Source: CAD feature listing. Evaluate the final solid. Frame: model axes, mm. Face numbers are marked on the shaded views. A direction names the side the tool comes from. Round coordinates to 2 decimals unless told otherwise and drop trailing zeros. Loops run counter-clockwise (first coordinate to the right, second up) from the corner with the lowest first, then second, coordinate; pieces in that order, holes last. Notation, with made-up numbers: M 65.5,56.5 L 79.5,56.5 A26 ccw 79.5,74.5 Z; hole C -19,9.25 d4. An arc over 180 degrees is marked long. Write each question's results on one line, items separated by ' | '. Start each with the question number.
1. Contact query for a flat-ended pin moving along its axis: pin 1 Ø4 at (x, z) = (-1, -13.5) entering from -Y. Output: stop coordinate, or through.
2. Set-up query: the marked faces 4 and 5. Return all of +Z, -Z, +X, -X, +Y, -Y with unobstructed straight access to the full face (end or side cutting, diameter ignored); none if empty.
3. Section C-C on y = 7.5. Output: boundary loops of the cut face in (x, z), and give its area (3 significant figures).
4. Ray query, line 1 (Z direction, x = 1.5, y = 0); line 2 (X direction, y = 10.75, z = -15.5); line 3 (Z direction, x = -6, y = 2.25). Return the intervals inside material, ascending.
5. Section A-A on z = -15.5. Output: boundary loops of the cut face in (x, y).
6. Draft query along Z for the marked faces 1, 2 and 3. Return one class per face: released by +Z, released by -Z, zero draft, split by the parting line, or undercut.
7. Section D-D on x = -4.5. Output: boundary loops of the cut face in (y, z).
8. Section B-B on x = 0. Output: boundary loops of the cut face in (y, z), and give its area (3 significant figures).
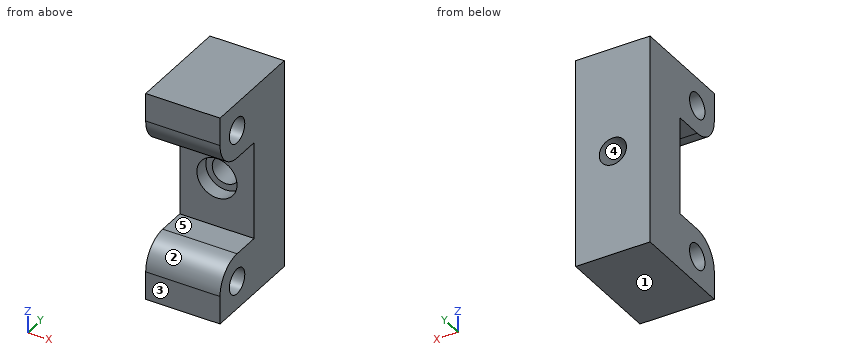
Autodesk Inventor part; units mm, degrees
ref_plane "Work Plane1" through (0, 5.5, 0) normal (0, 1, 0) x (-1, 0, 0)
ref_plane "YZ Plane" through (0, 0, 0) normal (1, 0, 0) x (0, 1, 0)
ref_plane "XY Plane" through (0, 0, 0) normal (0, 0, 1) x (1, 0, 0)
sketch "Sketch3" plane through (0, 0, 0) normal (1, 0, 0) x (0, 1, 0)
  circle A0 centre (0, 0) radius 5.65 construction
  line L0 (-5.65, 0) -> (-5.65, 5.65)
  line L1 (0, -5.65) -> (5.65, -5.65)
  arc A1 (-5.65, 0) -> (0, -5.65) centre (0, 0) ccw
  line L2 (-5.65, 5.65) -> (5.65, 5.65)
  line L3 (5.65, -15.5) -> (-5.65, -15.5) construction
  line L4 (5.65, 5.65) -> (15.65, 5.65)
  line L5 (15.65, 5.65) -> (15.65, -15.5)
  line L6 (5.65, -5.65) -> (5.65, -15.5)
  line L7 (15.65, -15.5) -> (5.65, -15.5) construction
  circle A2 centre (0, 0) radius 2.55
  line L8 (-5.65, -31) -> (-5.65, -36.65)
  arc A3 (0, -25.35) -> (-5.65, -31) centre (0, -31) ccw
  line L9 (0, -25.35) -> (5.65, -25.35)
  line L10 (-5.65, -36.65) -> (5.65, -36.65)
  line L11 (5.65, -36.65) -> (15.65, -36.65)
  line L12 (15.65, -36.65) -> (15.65, -15.5)
  line L13 (5.65, -25.35) -> (5.65, -15.5)
  circle A4 centre (0, -31) radius 2.55
  dimension "d19" = 11.3
  dimension "d20" = 5.65
  dimension "d23" = 10
  dimension "d24" = 10
  dimension "d25" = 11.3
  dimension "d26" = 5.1
  dimension "d36" = 21.15
ref_plane "Work Plane1" through (0, 5.5, 0) normal (0, 1, 0) x (-1, 0, 0)
extrude "Extrusion5" add sketch "Sketch3" along normal mid plane 15
sketch "Sketch5" plane through (0, 5.5, 0) normal (0, 1, 0) x (-1, 0, 0)
  line L0 (7.5, -25.35) -> (-7.5, -25.35) construction
  line L1 (-7.5, -5.65) -> (-7.5, -25.35) construction
  line L2 (-7.5, -5.65) -> (7.5, -5.65) construction
  line L3 (7.5, -25.35) -> (7.5, -5.65) construction
  line L4 (-7.5, -5.65) -> (-7.5, -25.35) construction
  line L5 (-7.5, -15.5) -> (7.5, -15.5) construction
  line L6 (-7.5, -5.65) -> (7.5, -5.65) construction
  line L7 (0, -5.65) -> (0, -25.35) construction
  circle A0 centre (0, -15.5) radius 4.05
  circle A1 centre (0, -15.5) radius 2.75
  point P0 (0, 0)
  dimension "d40" = 8.1
  dimension "d41" = 5.5
extrude "Extrusion6" cut sketch "Sketch5" along normal through all both and the other way through all contours A1
extrude "Extrusion7" cut sketch "Sketch5" along normal blind 3.1
properties part number "sostenedor_part2"
Taken from the geometry:
1) pin 1: y = 5.65
2) face 4: +Y, -Y | face 5: +X, -X, -Y
3) outline: M -7.5,-36.65 L 7.5,-36.65 L 7.5,5.65 L -7.5,5.65 Z; hole C 0,-15.5 d8.1 | area: 583 mm^2
4) line 1: -36.65 to -33.55, -28.45 to -25.35, -5.65 to -2.55, 2.55 to 5.65 | line 2: -7.5 to -2.75, 2.75 to 7.5 | line 3: -36.65 to -32.2, -29.8 to -25.35, -5.65 to -1.2, 1.2 to 5.65
5) outline: M -7.5,5.65 L -4.05,5.65 L -4.05,8.6 L -2.75,8.6 L -2.75,15.65 L -7.5,15.65 Z; M 2.75,8.6 L 4.05,8.6 L 4.05,5.65 L 7.5,5.65 L 7.5,15.65 L 2.75,15.65 Z
6) face 1: released by -Z | face 2: undercut | face 3: zero draft
7) outline: M -5.65,-36.65 L 15.65,-36.65 L 15.65,5.65 L -5.65,5.65 L -5.65,0 A5.65 ccw 0,-5.65 L 5.65,-5.65 L 5.65,-25.35 L 0,-25.35 A5.65 ccw -5.65,-31 Z; hole C 0,-31 d5.1; hole C 0,0 d5.1
8) outline: M -5.65,-36.65 L 15.65,-36.65 L 15.65,-18.25 L 8.6,-18.25 L 8.6,-19.55 L 5.65,-19.55 L 5.65,-25.35 L 0,-25.35 A5.65 ccw -5.65,-31 Z; M -5.65,0 A5.65 ccw 0,-5.65 L 5.65,-5.65 L 5.65,-11.45 L 8.6,-11.45 L 8.6,-12.75 L 15.65,-12.75 L 15.65,5.65 L -5.65,5.65 Z; hole C 0,-31 d5.1; hole C 0,0 d5.1 | area: 561 mm^2
